Input: part model. Units: mm. Frame: model coordinates. Face numbers are marked on the shaded views. A direction names the side the tool comes from. Round coordinates to 2 decimals unless told otherwise and drop trailing zeros. Loops run counter-clockwise (first coordinate to the right, second up) from the corner with the lowest first, then second, coordinate; pieces in that order, holes last. Notation, with made-up numbers: (-7, 30) -> (26, 30) arc R12 cw to (26, 46) -> close; hole circle Ø1 at (37, 19). An arc over 180 degrees is marked (long way). Answer in a Markdown table with one row per item. Add a question column.
Q1. Mould query, pull axis Y, two halves, no side actions, for the marked faces 1, 2 and 3. Classes: pulls with the +Y half, pulls with the -Y half, needs draft (parallel to the pull), parting line crosses it, or undercut.
Q2. Section D-D, the plane y = 57.5. Output: boundary loops of the cut face in (x, z).
Q3. Reachability of the marked faces 4, 5, 6 and 7 from +Z, -Z, +X, -X, +Y, -Y: full face, straight path, thin tool, end or side. Return the list, or none.
Q4. Section B-B, the plane x = -8.5. Give the number of separate pieces and of enclosed holes in the cut face, and give its area (3 significant figures).
Q5. Pin query (flat end, axial travel): pin 1 (1.4 mm diameter, centred on x = -29.5, y = 58, fed in from -Z); pin 2 (1.3 mm diameter, centred on y = 19.5, z = -4, fed in from -X); pin 3 (1 mm diameter, centred on y = 31, z = 7, fed in from -X). Return the tip coordinate at first contact, or that it passes through.
Q6. Section A-A, the plane y = 29. Output: boundary loops of the cut face in (x, z), and give its area (3 significant figures).
Q7. Section C-C, the plane y = 4. Output: boundary loops of the cut face in (x, z), and give its area (3 significant figures).
Q8. Ray query, L1, parallel to Y at x = -14.5, z = -19; L2, parallel to X at y = 16.8, z = 0; L3, parallel to Z at x = -1, y = 24.5. Return the intervals inside material, ascending. Write a range as from..to.
```python
from build123d import *

# Parameters (mm, degrees)
CUT_EXTRUDE1_DEPTH  = 5
CUT_EXTRUDE3_DEPTH  = 45
SKETCH8_R           = 40
CUT_EXTRUDE4_DEPTH  = 32
SKETCH9_R           = 32
SKETCH9_R_2         = 24.5
CUT_EXTRUDE5_DEPTH  = 14
SKETCH10_R          = 26
CUT_EXTRUDE6_DEPTH  = 14
FILLET1_R           = 7
FILLET2_R           = 7
CUT_REVOLVE1_START  = 22
CUT_REVOLVE1_DEPTH  = 30.5
CUT_EXTRUDE12_DEPTH = 5
SKETCH18_W          = 13
SKETCH18_H          = 8
CUT_EXTRUDE13_DEPTH = 5
SKETCH20_W          = 84
SKETCH20_H          = 7
CUT_EXTRUDE15_DEPTH = 5
SKETCH19_R          = 1.35
CUT_EXTRUDE14_DEPTH = 8


# Read off the part's stored shape, not the designer's step: Cut-Revolve1
with BuildPart() as part:
    # Sketch1 → Revolve1 (revolve)
    with BuildSketch(Plane.XY, mode=Mode.PRIVATE) as revolve1_sk:
        with BuildLine():
            Line((22.5, 0), (32, 0))
            ThreePointArc((32, 0), (33.414213562, 0.585786438), (34, 2))
            Line((34, 2), (34, 18))
            Line((34, 18), (40, 18))
            ThreePointArc((40, 18), (41.414213562, 18.585786438), (42, 20))
            Line((42, 20), (42, 55))
            ThreePointArc((42, 55), (40.535533906, 58.535533906), (37, 60))
            Line((37, 60), (0, 60))
            Line((0, 60), (0, 18))
            Line((0, 18), (22.5, 18))
            Line((22.5, 18), (22.5, 0))
        make_face()
    revolve(revolve1_sk.sketch.rotate(Axis((0, 2, 0), (0, 1, 0)), 90), axis=Axis((0, 2, 0), (0, 1, 0)))

    # Sketch5 → Cut-Extrude1 (cut)
    with BuildSketch(Plane(origin=(0, 60, 0), x_dir=(1, 0, 0), z_dir=(0, 1, 0))):
        with BuildLine():
            Line((-42, 0), (-40, 0))
            Line((-40, 0), (40, 0))
            Line((40, 0), (42, 0))
            ThreePointArc((42, 0), (0, 42), (-42, 0))
        make_face()
    extrude(amount=-CUT_EXTRUDE1_DEPTH, mode=Mode.SUBTRACT)

    # Sketch7 → Cut-Extrude3 (cut)
    with BuildSketch(Plane.XZ.offset(-18)):
        with BuildLine():
            Line((-21, 0), (21, 0))
            ThreePointArc((21, 0), (0, -21), (-21, 0))
        make_face()
    extrude(amount=-CUT_EXTRUDE3_DEPTH, mode=Mode.SUBTRACT)

    # Sketch8 → Cut-Extrude4 (cut)
    with BuildSketch(Plane(origin=(0, 52.5, 0), x_dir=(1, 0, 0), z_dir=(0, 1, 0))):
        with Locations(Location((0, 0, 0), (0, 0, 270))):
            Circle(SKETCH8_R)
        with BuildLine():
            Line((22.912878475, -2), (-22.912878475, -2))
            ThreePointArc((-22.912878475, -2), (0, 23), (22.912878475, -2))
        make_face(mode=Mode.SUBTRACT)
    extrude(amount=-CUT_EXTRUDE4_DEPTH, mode=Mode.SUBTRACT)

    # Sketch9 → Cut-Extrude5 (cut)
    with BuildSketch(Plane(origin=(0, 2, 0), x_dir=(-1, 0, 0), z_dir=(0, -1, 0))):
        with Locations(Location((0, 0, 0), (0, 0, 90))):
            Circle(SKETCH9_R)
        with Locations(Location((0, 0, 0), (0, 0, 90))):
            Circle(SKETCH9_R_2, mode=Mode.SUBTRACT)
    extrude(amount=-CUT_EXTRUDE5_DEPTH, mode=Mode.SUBTRACT)

    # Sketch10 → Cut-Extrude6 (cut)
    with BuildSketch(Plane(origin=(0, 2, 0), x_dir=(-1, 0, 0), z_dir=(0, -1, 0))):
        Circle(SKETCH10_R)
    extrude(amount=-CUT_EXTRUDE6_DEPTH, mode=Mode.SUBTRACT)

    # Fillet1
    fillet1_edges = [part.edges().sort_by_distance(p)[0] for p in [
        (21, 36.5, 0),
        (-21, 36.5, 0),
    ]]
    fillet(fillet1_edges, radius=FILLET1_R)

    # Fillet2
    fillet2_edges = [part.edges().sort_by_distance(p)[0] for p in [
        (-22.912878475, 36.5, 2),
        (22.912878475, 36.5, 2),
    ]]
    fillet(fillet2_edges, radius=FILLET2_R)

    # Cut-Revolve1 outline → Cut-Revolve1 (cut)
    with BuildSketch(Plane(origin=(0, 0, 0), x_dir=(1, 0, 0), z_dir=(0, 1, 0)).offset(CUT_REVOLVE1_START)):
        with BuildLine():
            Line((-34.641016151, -20), (-36.373066959, -21))
            ThreePointArc((-36.373066959, -21), (0, -42), (36.373066959, -21))
            Line((36.373066959, -21), (34.641016151, -20))
            ThreePointArc((34.641016151, -20), (0, -40), (-34.641016151, -20))
        make_face()
    extrude(amount=CUT_REVOLVE1_DEPTH, mode=Mode.SUBTRACT)

    # Sketch15 → Cut-Extrude12 (cut)
    with BuildSketch(Plane(origin=(0, 20.5, 0), x_dir=(1, 0, 0), z_dir=(0, 1, 0))):
        with BuildLine():
            Line((-28.124355653, -3.514579578), (-26.124355653, -3.514579578))
            ThreePointArc((-26.124355653, -3.514579578), (-24.710142091, -2.928793141), (-24.124355653, -1.514579578))
            Line((-24.124355653, -1.514579578), (-24.124355653, 8.485420422))
            ThreePointArc((-24.124355653, 8.485420422), (-24.710142091, 9.899633984), (-26.124355653, 10.485420422))
            Line((-26.124355653, 10.485420422), (-28.124355653, 10.485420422))
            ThreePointArc((-28.124355653, 10.485420422), (-29.538569215, 9.899633984), (-30.124355653, 8.485420422))
            Line((-30.124355653, 8.485420422), (-30.124355653, -1.514579578))
            ThreePointArc((-30.124355653, -1.514579578), (-29.538569215, -2.928793141), (-28.124355653, -3.514579578))
        make_face()
    extrude(amount=-CUT_EXTRUDE12_DEPTH, mode=Mode.SUBTRACT)

    # Sketch18 → Cut-Extrude13 (cut)
    with BuildSketch(Plane(origin=(0, 55, 0), x_dir=(1, 0, 0), z_dir=(0, 1, 0))):
        with Locations((0.796512215, 32.951769165)):
            Rectangle(SKETCH18_W, SKETCH18_H)
    extrude(amount=-CUT_EXTRUDE13_DEPTH, mode=Mode.SUBTRACT)

    # Sketch20 → Cut-Extrude15 (cut)
    with BuildSketch(Plane(origin=(0, 60, 0), x_dir=(1, 0, 0), z_dir=(0, 1, 0))):
        with Locations((0, -3.5)):
            Rectangle(SKETCH20_W, SKETCH20_H)
    extrude(amount=-CUT_EXTRUDE15_DEPTH, mode=Mode.SUBTRACT)

    # Sketch19 → Cut-Extrude14 (cut)
    with BuildSketch(Plane(origin=(0, 0, 7), x_dir=(-1, 0, 0), z_dir=(0, 0, -1))):
        with Locations((0, 57.5)):
            Circle(SKETCH19_R)
        with Locations((-29.412558482, 57.5)):
            Circle(SKETCH19_R)
        with Locations((29.412558482, 57.5)):
            Circle(SKETCH19_R)
    extrude(amount=-CUT_EXTRUDE14_DEPTH, mode=Mode.SUBTRACT)


solid = part.part
```
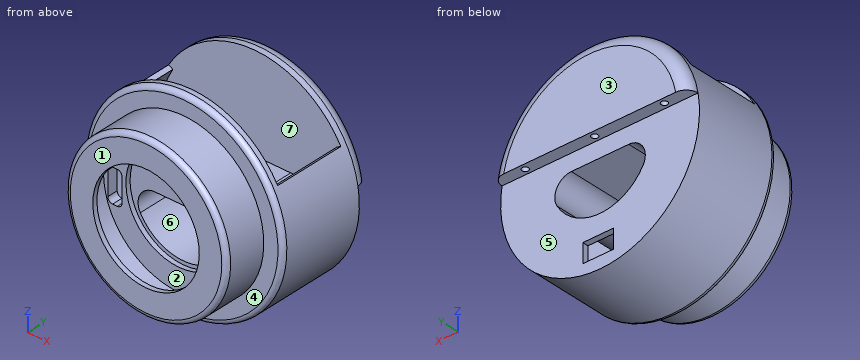
Answer block:
| question | item | result |
|---|---|---|
| 1 | face 1 | pulls with the -Y half |
| 1 | face 2 | undercut |
| 1 | face 3 | pulls with the +Y half |
| 2 | outline | (-40.73, 7) -> (-30.76, 7) -> (-30.76, 15) -> (-28.06, 15) -> (-28.06, 7) -> (-1.35, 7) -> (-1.35, 15) -> (1.35, 15) -> (1.35, 7) -> (28.06, 7) -> (28.06, 15) -> (30.76, 15) -> (30.76, 7) -> (40.73, 7) arc R41.33 ccw to start |
| 3 | face 4 | -Y |
| 3 | face 5 | -Z, +X, -X, +Y |
| 3 | face 6 | +Y, -Y |
| 3 | face 7 | none |
| 4 | separate pieces | 2 |
| 4 | enclosed holes | 1 |
| 4 | area | 833 mm^2 |
| 5 | pin 1 | z = 15 |
| 5 | pin 2 | x = -41.85 |
| 5 | pin 3 | x = -41.49 |
| 6 | outline | (-36.37, 21) arc R42 ccw (long way) to (36.37, 21) -> (34.64, 20) arc R40 cw (long way) to (-34.64, 20) -> close; (-21.85, -7.19) arc R23 ccw to (21.85, -7.19) arc R7 ccw to (15.2, 2) -> (-15.2, 2) arc R7 ccw to start; hole (-18.19, -10.5) arc R21 ccw to (18.19, -10.5) arc R7 ccw to (12.12, 0) -> (-12.12, 0) arc R7 ccw to start |
| 6 | area | 586 mm^2 |
| 7 | outline | circle Ø68 at (0, 0); hole circle Ø64 at (0, 0) |
| 7 | area | 415 mm^2 |
| 8 | L1 | 0..2, 16..20.5, 52.5..55 |
| 8 | L2 | -34..-30.12, -24.12..-22.5, 22.5..34 |
| 8 | L3 | -41.99..-39.99, -22.98..-20.98, 0..2 |
